```python
from build123d import *

# Parameters (mm, degrees)
F0_W      = 69.85
F0_H      = 44.45
F1_DEPTH  = 3.175
F2_R      = 25.4
F3_R      = 5.08
F4_W      = 10.16
F4_H      = 12.7
F5_DEPTH  = 25.4
F6_R      = 3.81
F7_DEPTH  = 19.05
F8_R      = 5.07999
F9_R      = 10.795
F10_DEPTH = 3.175
F11_R     = 0.8255
F12_W     = 27.94
F12_H     = 27.94
F12_W_2   = 25.4
F12_H_2   = 25.4
F13_DEPTH = 1.27


# Not quite as in the source:
# - a fillet or chamfer is up to 0.001 mm smaller than in the source, because OpenCascade refuses the exact size


with BuildPart() as f1:
    # F0 (on Front) → F1 (new body)
    with BuildSketch(Plane.XZ):
        with Locations((0, 22.225)):
            Rectangle(F0_W, F0_H)
    extrude(amount=F1_DEPTH)

    # F2
    f2_edges = [f1.edges().sort_by_distance(p)[0] for p in [
        (-34.925, -1.5875, 44.45),
        (34.925, -1.5875, 44.45),
    ]]
    fillet(f2_edges, radius=F2_R)

    # F3
    f3_edges = [f1.edges().sort_by_distance(p)[0] for p in [
        (-34.925, -1.5875, 0),
        (34.925, -1.5875, 0),
    ]]
    fillet(f3_edges, radius=F3_R)

    # F4 (on face) → F5 (join)
    with BuildSketch(Plane(origin=(0, 0, 0), x_dir=(1, 0, 0), z_dir=(0, 0, -1))):
        with Locations((0, -6.35)):
            Rectangle(F4_W, F4_H)
    extrude(amount=-F5_DEPTH)

    # F6 (on face) → F7 (cut)
    with BuildSketch(Plane(origin=(0, 0, 0), x_dir=(1, 0, 0), z_dir=(0, 0, -1))):
        with Locations((0, -6.35)):
            Circle(F6_R)
    extrude(amount=-F7_DEPTH, mode=Mode.SUBTRACT)

    # F8 (radius 5.08 in the source; OpenCascade refuses exactly that, so slightly less here)
    f8_edges = [f1.edges().sort_by_distance(p)[0] for p in [
        (-5.08, 12.7, 12.7),
        (5.08, 12.7, 12.7),
        (0, 0, 25.4),
        (-5.08, 6.35, 25.4),
        (0, 12.7, 25.4),
        (5.08, 6.35, 25.4),
        (5.08, 0, 12.7),
        (-5.08, 0, 12.7),
    ]]
    fillet(f8_edges, radius=F8_R)

    # F9 (on face) → F10 (join)
    with BuildSketch(Plane(origin=(0, 0, 0), x_dir=(1, 0, 0), z_dir=(0, 0, -1))):
        with BuildLine():
            Line((-5.08, 6.35), (-5.08, 3.175))
            Line((-5.08, 3.175), (5.08, 3.175))
            Line((5.08, 3.175), (5.08, 6.35))
            ThreePointArc((5.08, 6.35), (0, 33.3336274728), (-5.08, 6.35))
        make_face()
        with Locations((0, 19.3636274728)):
            Circle(F9_R, mode=Mode.SUBTRACT)
    extrude(amount=-F10_DEPTH)

    # F11
    f11_edges = [f1.edges().sort_by_distance(p)[0] for p in [
        (-10.795, -19.363627, 3.175),
        (0, -33.333627, 3.175),
        (0, -33.333627, 0),
        (-10.795, -19.363627, 0),
    ]]
    fillet(f11_edges, radius=F11_R)

    # F12 (on face) → F13 (cut)
    with BuildSketch(Plane.XZ.offset(3.175)):
        with Locations((0, 17.145)):
            Rectangle(F12_W, F12_H)
        with Locations((0, 17.145)):
            Rectangle(F12_W_2, F12_H_2, mode=Mode.SUBTRACT)
    extrude(amount=-F13_DEPTH, mode=Mode.SUBTRACT)


solid = f1.part
```
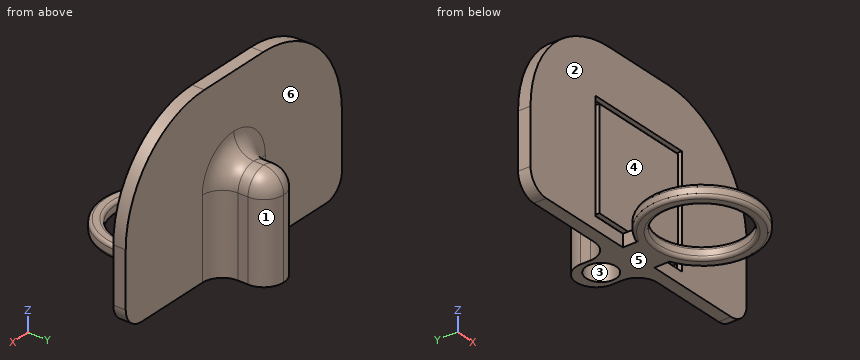
For this review, take the finished solid that the model builds, in its own axes (mm). Face numbers are marked on the shaded views. A direction names the side the tool comes from. Coordinates: 2 decimals unless noted, no trailing zeros.
1. Mouldability with a two-part tool opening along X and no side actions: class the marked faces 1, 2 and 3 as +X half, -X half, draft (parallel to the pull), parting line (faces both ways), or undercut.
2. For the marked faces 4, 5 and 6, list the 3-axis set-ups (+Z, -Z, +X, -X, +Y, -Y) from which the entire face can be reached by the end or side of a thin tool; tool diameter is ignored.
3. Insertion check: P1, Ø1, axis at y = -5, z = 1.5, coming from the -X side; P2, Ø6, axis at x = 23, z = 38.5, coming from the +Y side; P3, Ø3.5, axis at y = -6, z = 2, coming from the +X side; P4, Ø12, axis at y = -12, z = 31.5, coming from the -X side. Each pin has a flat end and moves straight along its axis. Give the tip position at first contact, or say it passes through.
4. For line 1 (Y direction, x = 0, z = 1.35); line 2 (Z direction, x = 6, y = -3) (3 decimals); line 3 (X direction, y = -3, z = 7) (3 decimals), list the stretches that pass through material, from the lowest coordinate up.
5. Add section B-B, the plane x = -8. Count the separate pieces of the cut face and the enclosed holes in it, then the cut area to 3 significant figures.
Result:
1. face 1: +X half
1. face 2: draft
1. face 3: undercut
2. face 4: +Z, +X, -X, -Y
2. face 5: -Z, +X, -X, +Y, -Y
2. face 6: +Z, +Y
3. P1: stops at x = -5.08
3. P2: stops at y = 0
3. P3: stops at x = 7.76
3. P4: passes through
4. line 1: y = -33.33 to -30.16, -8.57 to 2.54, 10.16 to 12.7
4. line 2: z = 0 to 3.175, 4.445 to 29.845, 31.115 to 44.45
4. line 3: x = -34.925 to -13.97, -12.7 to 12.7, 13.97 to 34.925
5. separate pieces: 3
5. enclosed holes: 0
5. area: 174 mm2
